For this review, take the finished solid that the model builds, in its own axes (mm). Give positions to 0.01 mm unless a question says otherwise; leave off trailing zeros. Write each loop counter-clockwise with the first axis right and the second up, starting at its lowest first coordinate (ties: lowest second). Pieces come first, ordered by that corner, then holes.
1) For P1, Ø3, axis at x = 30, y = 6, coming from the -Z side, flat-tipped, find the tip position at first contact; note if it passes through.
2) We need section D-D on x = 5.5. Give the boundary of the cut face in (y, z), and give its area (3 significant figures).
3) We need section A-A on y = 80. Give the boundary of the cut face in (x, z).
4) Wall thickness on line 1 along Y through (x, z) = (6, 4.7); line 2 along X through (y, z) = (142, 4.55); line 3 along Y through (x, z) = (33, 5.2): over which ranges is each line inside the solid? List them lowest first.
5) We need section C-C on z = 4.7. Give the number of separate pieces and of enclosed holes in the cut face, and give its area (3 significant figures).
6) We need section B-B on x = 18. Give the boundary of the cut face in (y, z), and give its area (3 significant figures).
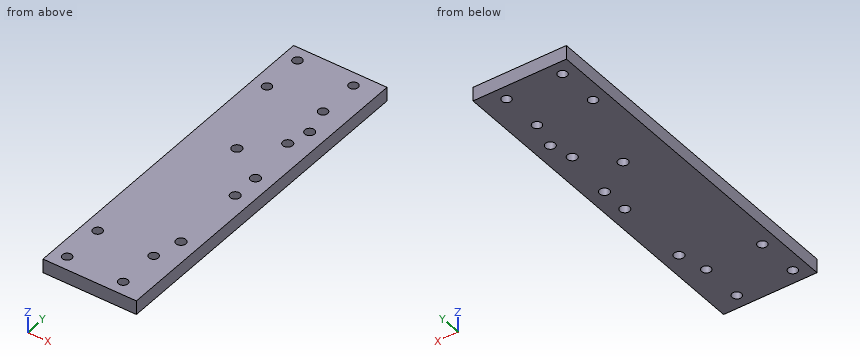
from build123d import *

# Parameters (mm, degrees)
F0_W     = 40
F0_H     = 148
F0_R     = 2
F0_R_2   = 2.1
F1_DEPTH = 6


with BuildPart() as f1:
    # F0 (on Top) → F1 (new body)
    with BuildSketch(Plane.XY):
        with Locations((20, 74)):
            Rectangle(F0_W, F0_H)
        with Locations((6, 6)):
            Circle(F0_R, mode=Mode.SUBTRACT)
        with Locations((6, 24)):
            Circle(F0_R, mode=Mode.SUBTRACT)
        with Locations((30, 6)):
            Circle(F0_R, mode=Mode.SUBTRACT)
        with Locations((30, 24)):
            Circle(F0_R, mode=Mode.SUBTRACT)
        with Locations((33, 36)):
            Circle(F0_R_2, mode=Mode.SUBTRACT)
        with Locations((33, 68)):
            Circle(F0_R_2, mode=Mode.SUBTRACT)
        with Locations((18, 89.69)):
            Circle(F0_R_2, mode=Mode.SUBTRACT)
        with Locations((6, 124)):
            Circle(F0_R, mode=Mode.SUBTRACT)
        with Locations((6, 142)):
            Circle(F0_R, mode=Mode.SUBTRACT)
        with Locations((33, 80)):
            Circle(F0_R_2, mode=Mode.SUBTRACT)
        with Locations((30.62, 102.31)):
            Circle(F0_R_2, mode=Mode.SUBTRACT)
        with Locations((33, 112)):
            Circle(F0_R_2, mode=Mode.SUBTRACT)
        with Locations((30, 124)):
            Circle(F0_R, mode=Mode.SUBTRACT)
        with Locations((30, 142)):
            Circle(F0_R, mode=Mode.SUBTRACT)
    extrude(amount=F1_DEPTH)


solid = f1.part
Results list:
1. P1: passes through
2. outline: (0, 0) - (4.06, 0) - (4.06, 6) - (0, 6) - close; (7.94, 0) - (22.06, 0) - (22.06, 6) - (7.94, 6) - close; (25.94, 0) - (122.06, 0) - (122.06, 6) - (25.94, 6) - close; (125.94, 0) - (140.06, 0) - (140.06, 6) - (125.94, 6) - close; (143.94, 0) - (148, 0) - (148, 6) - (143.94, 6) - close
2. area: 795 mm2
3. outline: (0, 0) - (30.9, 0) - (30.9, 6) - (0, 6) - close; (35.1, 0) - (40, 0) - (40, 6) - (35.1, 6) - close
4. line 1: y = 0 to 4, 8 to 22, 26 to 122, 126 to 140, 144 to 148
4. line 2: x = 0 to 4, 8 to 28, 32 to 40
4. line 3: y = 0 to 33.9, 38.1 to 65.9, 70.1 to 77.9, 82.1 to 109.9, 114.1 to 148
5. separate pieces: 1
5. enclosed holes: 14
5. area: 5,740 mm2
6. outline: (0, 0) - (87.59, 0) - (87.59, 6) - (0, 6) - close; (91.79, 0) - (148, 0) - (148, 6) - (91.79, 6) - close
6. area: 863 mm2
